The listing builds one solid part. Answer for the finished solid, in the listing's coordinates (mm). A direction names the side the tool comes from. Give positions to 0.01 mm unless a question says otherwise; leave off trailing zeros. Order: outer loops, then holes, each group sorted by start corner. A loop starts at its lowest first (then second) coordinate and runs counter-clockwise, first axis right, second up. Notation, with made-up numbers: (-9, 85) - (49, 85) arc R16 cw to (49, 91) - close; hole circle Ø6 at (30.5, 60.25). An arc over 180 degrees is marked (long way). Use CSV: the item, a comma, the result in double quotes.
```python
from build123d import *

# Parameters (mm, degrees)
SKETCH_2_W          = 50
SKETCH_2_H          = 5
EXTRUDE_1_DEPTH     = 5
SKETCH_3_R          = 2
CUT_EXTRUDE_1_DEPTH = 5
SKETCH_4_R          = 2
EXTRUDE_2_DEPTH     = 8


with BuildPart() as part:
    # 草图2 → 凸台-拉伸1 (new body)
    with BuildSketch(Plane.XY):
        with Locations((-16.04, 2.5)):
            Rectangle(SKETCH_2_W, SKETCH_2_H)
    extrude(amount=EXTRUDE_1_DEPTH)

    # 草图3 → 切除-拉伸1 (cut)
    with BuildSketch(Plane.XY.offset(5)):
        with Locations((-38.04, 2.5)):
            Circle(SKETCH_3_R)
    extrude(amount=-CUT_EXTRUDE_1_DEPTH, mode=Mode.SUBTRACT)

    # 草图4 → 凸台-拉伸2 (add)
    with BuildSketch(Plane.XY.offset(5)):
        with Locations((5.96, 2.5)):
            Circle(SKETCH_4_R)
    extrude(amount=EXTRUDE_2_DEPTH)


solid = part.part
```
Item 1: This flat-tipped pin is pushed along its axis until it touches: pin 1 (1.5 mm diameter, centred on x = -19.5, y = 3.5, fed in from +Z). Where does it stop, or does it pass through?
Taken from the geometry:
pin 1,"z = 5"
Item 2: The part is cut by section B-B (x = -38.04). Give the vertices of the cut face in (y, z).
Taken from the geometry:
outline,"(0, 0) - (0.5, 0) - (0.5, 5) - (0, 5) - close; (4.5, 0) - (5, 0) - (5, 5) - (4.5, 5) - close"
Item 3: The part is cut by section C-C (x = 5.96). Give the vertices of the cut face in (y, z), and give its area (3 significant figures).
Taken from the geometry:
outline,"(0, 0) - (5, 0) - (5, 5) - (4.5, 5) - (4.5, 13) - (0.5, 13) - (0.5, 5) - (0, 5) - close"
area,"57.0 mm^2"
Item 4: The part is cut by section D-D (z = 1.5). Give the vertices of the cut face in (x, y), and give its area (3 significant figures).
Taken from the geometry:
outline,"(-41.04, 0) - (8.96, 0) - (8.96, 5) - (-41.04, 5) - close; hole circle Ø4 at (-38.04, 2.5)"
area,"237 mm^2"
Item 5: Which of the six approach directions +Z, -Z, +X, -X, +Y, -Y give full straight-line access (tool end or side, diameter ignored) to faces 4 (the face through (4.373, 1.283, 8.944)), 5 (the face through (-41.04, 2, 2))?
Taken from the geometry:
face 4,"+Z"
face 5,"+Z, -Z, -X, +Y, -Y"
Item 6: The mould has two halves that part along Y. Classify faces 1 (the face through (-16, 0, 2)), 2 (the face through (8.96, 2, 2)), 3 (the face through (-36.193, 1.734, 2.535)): +Y half, -Y half, draft (parallel to the pull), parting line (faces both ways), or undercut.
Taken from the geometry:
face 1,"-Y half"
face 2,"draft"
face 3,"undercut"
Item 7: The part is cut by section A-A (y = 2.5). Give the vertices of the cut face in (x, z).
Taken from the geometry:
outline,"(-41.04, 0) - (-40.04, 0) - (-40.04, 5) - (-41.04, 5) - close; (-36.04, 0) - (8.96, 0) - (8.96, 5) - (7.96, 5) - (7.96, 13) - (3.96, 13) - (3.96, 5) - (-36.04, 5) - close"
Item 8: Find the intervals of material crossed by line 1 along Y through (x, z) = (-38.04, 3.3); line 2 along X through (y, z) = (2.6, 5.75); line 3 along Z through (x, y) = (-10.5, 4.1), in increasing order.
Taken from the geometry:
line 1,"0 to 0.5, 4.5 to 5"
line 2,"3.96 to 7.96"
line 3,"0 to 5"
